Geometry check sheet. Reference: the model listing, model coordinates, mm. A direction names the side the tool comes from. Round coordinates to 2 decimals unless told otherwise and drop trailing zeros. Order: outer loops, then holes, each group sorted by start corner. A loop starts at its lowest first (then second) coordinate and runs counter-clockwise, first axis right, second up. Notation, with made-up numbers: (22, 23) - (34, 23) arc R31 cw to (34, 51) - close; hole circle Ø2 at (28, 54.5). An arc over 180 degrees is marked (long way). Write each question's results on one line, items separated by ' | '.
```python
from build123d import *

# Parameters (mm, degrees)
SKETCH1_W                 = 98.79
SKETCH1_H                 = 44.78
BOSS_EXTRUDE1_DEPTH       = 30.05
SHELL1_T                  = -3
SHELL1_THICKNESS_2_FACE_W = 38.78
SHELL1_THICKNESS_2_FACE_H = 30.05
SHELL1_THICKNESS_2_DEPTH  = 7.95
SKETCH2_R                 = 1.75
CUT_EXTRUDE1_DEPTH        = 113.550944021
FILLET1_R                 = 2
CUT_EXTRUDE3_DEPTH        = 29.61
SKETCH5_R                 = 9
CUT_EXTRUDE4_DEPTH        = 20


with BuildPart() as part:
    # Sketch1 → Boss-Extrude1 (new body)
    with BuildSketch(Plane(origin=(0, 0, 0), x_dir=(1, 0, 0), z_dir=(0, 1, 0))):
        with Locations((49.395, 22.39)):
            Rectangle(SKETCH1_W, SKETCH1_H)
    extrude(amount=BOSS_EXTRUDE1_DEPTH)

    # Shell1
    shell1_openings = [part.faces().sort_by_distance(p)[0] for p in [
        (49.395, 30.05, -22.39),
        (49.395, 0, -22.39),
    ]]
    offset(amount=SHELL1_T, openings=shell1_openings, kind=Kind.INTERSECTION)

    # Shell1 thickness 2 face (on inner face of the shell) → Shell1 thickness 2 (add)
    with BuildSketch(Plane(origin=(3, 15.025, -22.39), x_dir=(0, 0, -1), z_dir=(-1, 0, 0))):
        Rectangle(SHELL1_THICKNESS_2_FACE_W, SHELL1_THICKNESS_2_FACE_H)
    extrude(amount=-SHELL1_THICKNESS_2_DEPTH)

    # Sketch2 → Cut-Extrude1 (cut, through all)
    with BuildSketch(Plane.XY):
        with Locations((77.08, 24.95)):
            Circle(SKETCH2_R)
        with Locations((77.08, 5.1)):
            Circle(SKETCH2_R)
        with Locations((47.36, 5.1)):
            Circle(SKETCH2_R)
        with Locations((47.36, 24.95)):
            Circle(SKETCH2_R)
    extrude(amount=-CUT_EXTRUDE1_DEPTH, mode=Mode.SUBTRACT)

    # Fillet1
    fillet1_edges = [part.edges().sort_by_distance(p)[0] for p in [
        (98.79, 30.05, -22.39),
        (0, 30.05, -22.39),
        (98.79, 0, -22.39),
        (0, 0, -22.39),
        (0, 15.025, -44.78),
        (98.79, 15.025, -44.78),
        (98.79, 15.025, 0),
        (0, 15.025, 0),
    ]]
    fillet(fillet1_edges, radius=FILLET1_R)

    # Sketch4 → Cut-Extrude3 (cut)
    with BuildSketch(Plane(origin=(98.79, 0, 0), x_dir=(0, 0, -1), z_dir=(1, 0, 0))):
        with BuildLine():
            Line((17.89, 30.05), (26.89, 30.05))
            Line((26.89, 30.05), (26.89, 13.05))
            ThreePointArc((26.89, 13.05), (26.011320344, 10.928679656), (23.89, 10.05))
            Line((23.89, 10.05), (20.89, 10.05))
            ThreePointArc((20.89, 10.05), (18.768679656, 10.928679656), (17.89, 13.05))
            Line((17.89, 13.05), (17.89, 30.05))
        make_face()
    extrude(amount=-CUT_EXTRUDE3_DEPTH, mode=Mode.SUBTRACT)

    # Sketch5 → Cut-Extrude4 (cut)
    with BuildSketch(Plane.ZY):
        with Locations((-22.39, 15.025)):
            Circle(SKETCH5_R)
    extrude(amount=-CUT_EXTRUDE4_DEPTH, mode=Mode.SUBTRACT)


solid = part.part
```
(1) Draft check along Y on faces 4 (the face through (97, 10.05, -22)), 5 (the face through (53, 15, -41.78)), 6 (the face through (32, 0, -2)), 7 (the face through (45.61, 5.18, -43.26)). Enter one of: released by +Y, released by -Y, zero draft, split by the parting line, or undercut.
Answers follow:
face 4: released by +Y | face 5: zero draft | face 6: released by -Y | face 7: undercut
(2) Depth check by flat-ended pin: pin 1 Ø4 at (x, y) = (47.36, 24.95) entering from -Z; pin 2 Ø3.5 at (x, z) = (97, -22) entering from +Y; pin 3 Ø4 at (y, z) = (10.5, -26) entering from -X. Enter the tip coordinate at first touch or a pass-through.
Answers follow:
pin 1: z = -44.78 | pin 2: y = 10.12 | pin 3: x = 95.79
(3) Access from +Z, -Z, +X, -X, +Y, -Y to the whole of each face (thin tool, end or side, straight path). Record for faces 1 (the face through (97, 21, -17.89)), 2 (the face through (53, 15, -3)), 3 (the face through (0.57, 15.24, -44.18)).
Answers follow:
face 1: +X, +Y | face 2: +Y, -Y | face 3: -Z, -X, +Y, -Y
(4) Section check B-B (z = -34). Record the cut outline in (x, y), then the cut area to 3 significant figures.
Answers follow:
outline: (0, 2) arc R2 ccw to (2, 0) - (10.95, 0) - (10.95, 30.05) - (2, 30.05) arc R2 ccw to (0, 28.05) - close; (95.79, 0) - (96.79, 0) arc R2 ccw to (98.79, 2) - (98.79, 28.05) arc R2 ccw to (96.79, 30.05) - (95.79, 30.05) - close | area: 416 mm²
(5) Section check D-D (y = 24.95). Give the number of separate pieces and of enclosed holes in the cut face, then the cut area to 3 significant figures.
Answers follow:
separate pieces: 5 | enclosed holes: 0 | area: 1,060 mm²
(6) Section check C-C (y = 5.1). Record the cut outline in (x, z).
Answers follow:
outline: (0, -42.78) arc R2 ccw to (2, -44.78) - (45.61, -44.78) - (45.61, -41.78) - (10.95, -41.78) - (10.95, -3) - (45.61, -3) - (45.61, 0) - (2, 0) arc R2 ccw to (0, -2) - close; (49.11, -44.78) - (75.33, -44.78) - (75.33, -41.78) - (49.11, -41.78) - close; (49.11, -3) - (75.33, -3) - (75.33, 0) - (49.11, 0) - close; (78.83, -44.78) - (96.79, -44.78) arc R2 ccw to (98.79, -42.78) - (98.79, -2) arc R2 ccw to (96.79, 0) - (78.83, 0) - (78.83, -3) - (95.79, -3) - (95.79, -41.78) - (78.83, -41.78) - close
(7) Section check A-A (x = 47.36). Record the cut outline in (y, z), then the cut area to 3 significant figures.
Answers follow:
outline: (0, -44.78) - (3.35, -44.78) - (3.35, -41.78) - (0, -41.78) - close; (0, -3) - (3.35, -3) - (3.35, 0) - (0, 0) - close; (6.85, -44.78) - (23.2, -44.78) - (23.2, -41.78) - (6.85, -41.78) - close; (6.85, -3) - (23.2, -3) - (23.2, 0) - (6.85, 0) - close; (26.7, -44.78) - (30.05, -44.78) - (30.05, -41.78) - (26.7, -41.78) - close; (26.7, -3) - (30.05, -3) - (30.05, 0) - (26.7, 0) - close | area: 138 mm²
(8) Material ranges on line 1 (X direction, y = 5, z = -43); line 2 (Y direction, x = 77.08, z = -1.7); line 3 (Z direction, x = 66, y = 28.5), recorded low to high.
Answers follow:
line 1: 0.01 to 45.61, 49.11 to 75.33, 78.83 to 98.78 | line 2: 0 to 3.35, 6.85 to 23.2, 26.7 to 30.05 | line 3: -44.78 to -41.78, -3 to 0
